Study the drawing (mm; zero at the part's minimum x, y, z) and answer. Coordinates: 2 decimals unless noted, no trailing zeros. Loops run counter-clockwise (first coordinate to the right, second up) from the corner with the lowest first, then second, coordinate; pieces in that order, holes last. Notation, with made-up numbers: (13.25, 73.5) - (59.25, 73.5) arc R24 cw to (59.25, 95.5) - close; hole circle Ø5 at (51.25, 78). An arc over 180 degrees is marked (long way). Use one line per item in the form item = value. Start each with the question number.
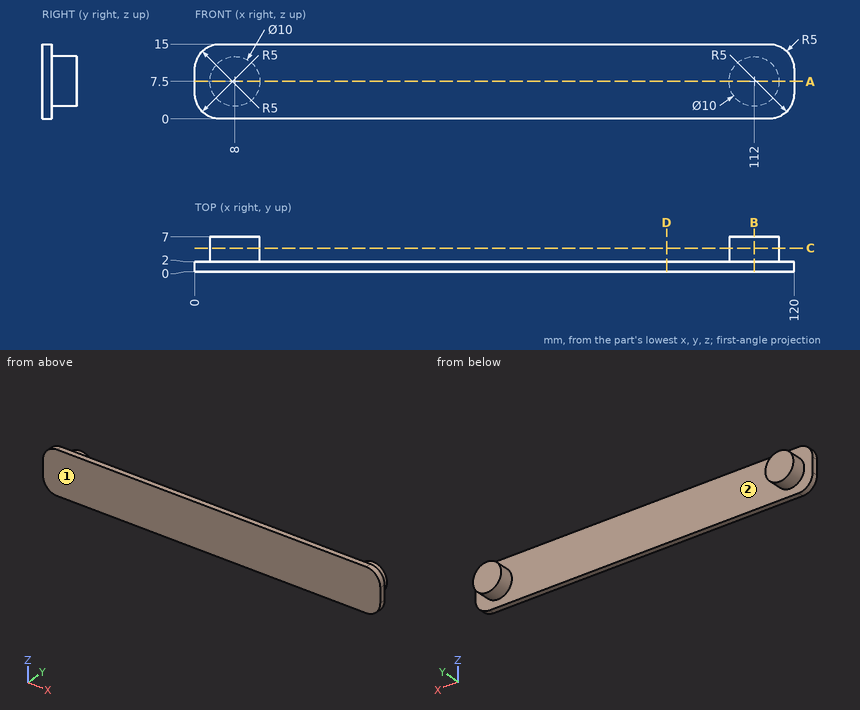
(1) A cutting plane is placed at C-C (y = 4.75). Determine the outline of the cut face in (x, z).
(2) A cutting plane is placed at D-D (x = 94.5). Determine the outline of the cut face in (y, z), then the cut area to 3 significant figures.
(3) Determine the mould class of the marked faces 1 and 2 for opening direction X: +X half, -X half, draft (parallel to the pull), parting line (faces both ways), or undercut.
(4) Each of these flat-tipped pins is pushed along its axis until it touches: pin 1 Ø2 at (y, z) = (5.5, 12) entering from +X; pin 2 Ø7.5 at (x, z) = (60, 8) entering from +Y. Where does it stop, or does it pass through?
(5) A cutting plane is placed at B-B (x = 112). Determine the outline of the cut face in (y, z), then the cut area to 3 significant figures.
(6) A cutting plane is placed at A-A (z = 7.5). Determine the outline of the cut face in (x, y), then the cut area to 3 significant figures.
(7) Find the intervals of material crossed by probe 1 along X at (y, z) = (4.25, 7.25); probe 2 along X at (y, z) = (3.5, 3.5); probe 3 along Y at (x, z) = (80, 6.75), in increasing order. Write a range as from..to.
Evaluation:
q1.outline = circle Ø10 at (8, 7.5); circle Ø10 at (112, 7.5)
q2.outline = (0, 0) - (2, 0) - (2, 15) - (0, 15) - close
q2.area = 30.0 mm^2
q3.face_1 = draft
q3.face_2 = undercut
q4.pin_1 = 115.57
q4.pin_2 = 2
q5.outline = (0, 0) - (2, 0) - (2, 2.5) - (7, 2.5) - (7, 12.5) - (2, 12.5) - (2, 15) - (0, 15) - close
q5.area = 80.0 mm^2
q6.outline = (0, 0) - (120, 0) - (120, 2) - (117, 2) - (117, 7) - (107, 7) - (107, 2) - (13, 2) - (13, 7) - (3, 7) - (3, 2) - (0, 2) - close
q6.area = 340 mm^2
q7.probe_1 = 3.01..12.99, 107.01..116.99
q7.probe_2 = 5..11, 109..115
q7.probe_3 = 0..2
